Autodesk Inventor part; units mm, degrees
ref_plane "Work Plane1" through (32.512, 0, -132.8293) normal (1, 0, 0) x (0, 1, 0)
ref_plane "XZ Plane" through (0, 0, 0) normal (0, 1, 0) x (-1, 0, 0)
ref_plane "XY Plane" through (0, 0, 0) normal (0, 0, 1) x (1, 0, 0)
sketch "Sketch1" plane through (0, 0, 0) normal (0, 1, 0) x (-1, 0, 0)
  line L0 (0, 0) -> (0, -394.9191)
  line L1 (0, 0) -> (32.512, 0)
  line L2 (32.512, 0) -> (32.512, -265.6586)
  line L3 (32.512, -265.6586) -> (0, -265.6586)
  dimension "d0" = 32.512
  dimension "d1" = 265.6586
revolve "Revolution1" add sketch "Sketch1" angle 360 about axis through (0, 0, 0) along (0, 0, -1)
fillet "Fillet1" radius 19.05 1 edges at (32.512, 0, -265.6586)
sketch "Sketch2" plane through (0, 0, 0) normal (1, 0, 0) x (0, 1, 0)
  line L0 (0, 0) -> (35.306, 0)
  line L1 (-32.512, 0) -> (32.512, 0)
  line L2 (35.306, 0) -> (35.306, 19.05)
  line L3 (35.306, 19.05) -> (0, 19.05)
  line L4 (0, 19.05) -> (0, 0)
  dimension "d4" = 35.306
  dimension "d5" = 19.05
revolve "Revolution2" add sketch "Sketch2" angle 360 about axis through (0, 0, 19.05) along (0, 0, -1)
fillet "Fillet2" radius 6.35 1 edges at (0, -35.306, 19.05)
sketch "Sketch3" plane through (0, 0, 0) normal (1, 0, 0) x (0, 1, 0)
  arc A0 (35.306, 12.7) -> (28.956, 19.05) centre (28.956, 12.7) ccw
  line L0 (32.267, 18.1184) -> (14.7581, 28.8176)
  line L1 (14.7581, 28.8176) -> (0, 28.8176)
  line L2 (0, 28.8176) -> (0, 19.05)
  line L3 (-28.956, 19.05) -> (28.956, 19.05)
  point P0 (0, 0)
revolve "Revolution3" add sketch "Sketch3" angle 360 about axis through (0, 0, 28.8176) along (0, 0, -1)
sketch "Sketch4" plane through (0, 0, 28.8176) normal (0, 0, 1) x (1, 0, 0)
  circle A0 centre (0, 0) radius 14.7581
extrude "Extrusion1" add sketch "Sketch4" along normal blind 3.6576
sketch "Sketch5" plane through (0, 0, -265.6586) normal (0, 0, -1) x (-1, 0, 0)
  circle A0 centre (0, 0) radius 13.462
extrude "Extrusion2" add sketch "Sketch5" along normal blind 8.1788
sketch "Sketch6" plane through (0, 0, 32.4752) normal (0, 0, 1) x (1, 0, 0)
  circle A0 centre (0, 0) radius 14.7581
  circle A1 centre (0, 0) radius 5.1761
extrude "Extrusion3" add sketch "Sketch6" along normal blind 2.54 contours A1
sketch "Sketch7" plane through (0, 0, -273.8374) normal (0, 0, -1) x (-1, 0, 0)
  circle A0 centre (0, 0) radius 5.1761
extrude "Extrusion4" add sketch "Sketch7" along normal blind 2.54
ref_plane "Work Plane1" through (32.512, 0, -132.8293) normal (1, 0, 0) x (0, 1, 0)
sketch "Sketch8" plane through (32.512, 0, -132.8293) normal (1, 0, 0) x (0, 1, 0)
  line L0 (25.1645, 74.2307) -> (25.1645, -47.9866) construction
  line L1 (25.1645, -47.9866) -> (-21.6706, -47.9866) construction
  line L2 (-21.6706, -47.9866) -> (-21.6706, 74.2307) construction
  line L3 (-21.6706, 74.2307) -> (25.1645, 74.2307) construction
  point P0 (0, 132.8293)
decal "Decal1"
properties part number "AVT-PP-35" material "Steel"
Design review of the part built by this model. Coordinates are the model's own, in mm. A direction names the side the tool comes from. Coordinates: 2 decimals unless noted, no trailing zeros. Loops run counter-clockwise (first coordinate to the right, second up) from the corner with the lowest first, then second, coordinate; pieces in that order, holes last. Notation, with made-up numbers: (17.5, -0.5) - (35.5, -0.5) arc R3 ccw to (35.5, 3.5) - close; hole circle Ø5 at (65.25, 42.25). An arc over 180 degrees is marked (long way). Use CSV: the item, a comma, the result in double quotes. Start each with the question number.
1) For pin 1 Ø1 at (y, z) = (-17, -202.5) entering from +X; pin 2 Ø1 at (x, y) = (-18, -18) entering from -Z; pin 3 Ø2 at (x, y) = (-5, -8.5) entering from +Z, all flat-tipped, find the tip position at first contact; note any pin that passes through.
2) Wall thickness on L1, parallel to Z at x = 6, y = -0.5; L2, parallel to Y at x = 3.5, z = -244; L3, parallel to X at y = 16, z = -173.5: over which ranges is each line inside the solid? List them lowest first. Write a range as from..to.
3) Consider section A-A on z = -87.5. Write out the cut boundary in (x, y).
4) Tool access review of faces 1 (the flat face through (0, -6, 32.475)), 2 (the cylindrical face through (34.466, -7.654, 6.439)), 3 (the cylindrical face through (10.683, 8.191, -269.691)): name each direction out of +Z, -Z, +X, -X, +Y, -Y from which nothing blocks a thin tool from reaching the whole face with its end or side.
Geometry says:
1,pin 1,"x = 28.01"
1,pin 2,"z = -261.8"
1,pin 3,"z = 32.48"
2,L1,"-273.84..32.48"
2,L2,"-32.32..32.32"
2,L3,"-28.3..28.3"
3,outline,"circle Ø65.02 at (0, 0)"
4,face 1,"+Z"
4,face 2,"+Z, -Z"
4,face 3,"-Z"
